Can you work these out from the model? Positions are in its coordinate system, mm. Face numbers are marked on the shaded views. A direction names the side the tool comes from. Give positions to 0.01 mm unless a question says otherwise; leave off trailing zeros. Order: outer loops, then holes, each group sorted by start corner. A loop starts at its lowest first (then second) coordinate and runs counter-clockwise, first axis right, second up. Notation, with made-up numbers: (73.25, 6.5) - (115.25, 6.5) arc R32 cw to (115.25, 35.5) - close; hole circle Ø9 at (-32.75, 70). An arc over 180 degrees is marked (long way). Answer as a JSON object with one key per item and string values.
```python
from build123d import *

# Parameters (mm, degrees)
SKETCH1_R           = 8.5
BOSS_EXTRUDE1_DEPTH = 5.5
SKETCH10_R          = 2.485
BOSS_EXTRUDE3_DEPTH = 13.5
SKETCH12_R          = 4.5
CUT_EXTRUDE4_DEPTH  = 2.54
CHAMFER2_SIZE       = 0.5
SKETCH14_R          = 2.04
CUT_EXTRUDE5_DEPTH  = 2.35
SKETCH15_R          = 1.065
CUT_EXTRUDE6_DEPTH  = 19.076227483
SKETCH16_R          = 5
CUT_EXTRUDE7_DEPTH  = 10
CIRPATTERN1_COUNT   = 3


with BuildPart() as part:
    # Sketch1 → Boss-Extrude1 (new body)
    with BuildSketch(Plane(origin=(0, 0, 0), x_dir=(1, 0, 0), z_dir=(0, 1, 0))):
        with Locations(Location((0, 0, 0), (0, 0, 270))):
            Circle(SKETCH1_R)
    extrude(amount=-BOSS_EXTRUDE1_DEPTH)

    # Sketch10 → Boss-Extrude3 (add)
    with BuildSketch(Plane(origin=(0, 0, 0), x_dir=(1, 0, 0), z_dir=(0, 1, 0))):
        with Locations(Location((0, 0, 0), (0, 0, 270))):
            Circle(SKETCH10_R)
    extrude(amount=BOSS_EXTRUDE3_DEPTH)

    # Sketch12 → Cut-Extrude4 (cut)
    with BuildSketch(Plane.XZ.offset(5.5)):
        with Locations(Location((0, 0, 0), (0, 0, 270))):
            Circle(SKETCH12_R)
    extrude(amount=-CUT_EXTRUDE4_DEPTH, mode=Mode.SUBTRACT)

    # Chamfer2
    chamfer2_edges = [part.edges().sort_by_distance(p)[0] for p in [
        (0, 13.5, -2.485),
    ]]
    chamfer(chamfer2_edges, length=CHAMFER2_SIZE)

    # Sketch14 → Cut-Extrude5 (cut)
    with BuildSketch(Plane(origin=(0, 0, 0), x_dir=(1, 0, 0), z_dir=(0, 1, 0))):
        with Locations(Location((0, -5.7605, 0), (0, 0, 270))):
            Circle(SKETCH14_R)
        with Locations(Location((-5.033935185, 2.880072698, 0), (0, 0, 270))):
            Circle(SKETCH14_R)
        with Locations(Location((4.965987867, 2.919302101, 0), (0, 0, 270))):
            Circle(SKETCH14_R)
    extrude(amount=-CUT_EXTRUDE5_DEPTH, mode=Mode.SUBTRACT)

    # Sketch15 → Cut-Extrude6 (cut, through all)
    with BuildSketch(Plane(origin=(0, 0, 0), x_dir=(1, 0, 0), z_dir=(0, 1, 0))):
        with Locations(Location((4.965987867, 2.919302101, 0), (0, 0, 270))):
            Circle(SKETCH15_R)
        with Locations(Location((-5.033935185, 2.880072698, 0), (0, 0, 270))):
            Circle(SKETCH15_R)
        with Locations(Location((0, -5.7605, 0), (0, 0, 270))):
            Circle(SKETCH15_R)
    extrude(amount=-CUT_EXTRUDE6_DEPTH, mode=Mode.SUBTRACT)

    # Sketch16 → Cut-Extrude7 (cut)
    with BuildSketch(Plane(origin=(0, 0, 0), x_dir=(-1, 0, 0), z_dir=(0, 0.7071067811865475, -0.7071067811865477))):
        with Locations((0, -12.01040764)):
            Circle(SKETCH16_R)
    cut_extrude7 = extrude(amount=CUT_EXTRUDE7_DEPTH, mode=Mode.SUBTRACT)

    # CirPattern1: Cut-Extrude7 ×3 about axis
    cirpattern1_axis = Axis((0, 0, 0), (0, 1, 0))
    for i in range(1, CIRPATTERN1_COUNT):
        add(cut_extrude7.rotate(cirpattern1_axis, i * 360 / CIRPATTERN1_COUNT), mode=Mode.SUBTRACT)


solid = part.part
```
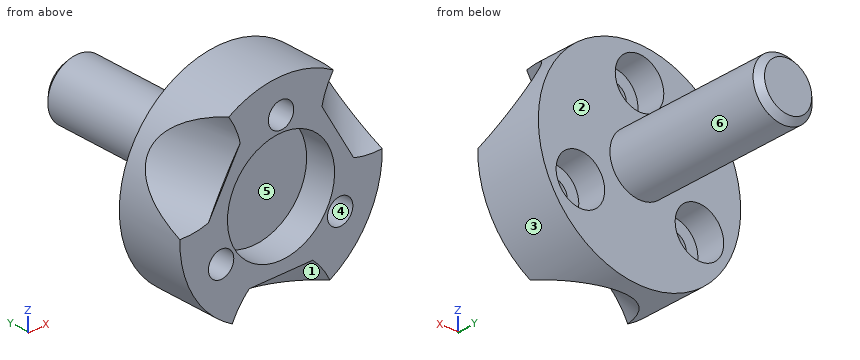
Q1. If we section it at B-B, the plane y = 2.5: Please give me the cut outline in (x, z) (3 decimals), then the cut area to 3 significant figures.
Recorded:
{"outline": "circle Ø4.97 at (0, 0)", "area": "19.4 mm^2"}
Q2. I need wall thicknesses on L1, parallel to X at y = -3.75, z = -2.75; L2, parallel to Y at x = -7.5, z = -1.25; L3, parallel to Y at x = 0.25, z = 3.25. Which ranges of each line are inside material? Lowest first, please.
Recorded:
{"L1": "x = -8.04 to -6.09, -3.98 to -3.56, 3.56 to 3.91, 6.02 to 8.04", "L2": "y = -5.5 to 0", "L3": "y = -2.96 to 0"}
Q3. We'd pull the mould along X, two halves only. Please class the marked faces 1, 2 and 3: released by +X, released by -X, zero draft, split by the parting line, or undercut.
Recorded:
{"face 1": "undercut", "face 2": "zero draft", "face 3": "split by the parting line"}
Q4. Which directions (+Z, -Z, +X, -X, +Y, -Y) give clear straight access to the entire face, cutting with the end or side of a thin tool? Please do the marked faces 4, 5 and 6.
Recorded:
{"face 4": "+Y, -Y", "face 5": "-Y", "face 6": "+Y"}
Q5. I'm going to push flat-ended pins straight in: pin 1 Ø3 at (x, y) = (3, 0.5) entering from -Z; pin 2 Ø5 at (y, z) = (3.5, 3.5) entering from +X; pin 3 Ø10 at (y, z) = (-3, -1.5) entering from -X; pin 4 Ø3 at (x, z) = (4.97, -2.92) entering from +Y. Where does each tip first touch, or does it pass through?
Recorded:
{"pin 1": "stops at z = -8.35", "pin 2": "stops at x = 2.27", "pin 3": "stops at x = -8.5", "pin 4": "stops at y = -2.35"}
